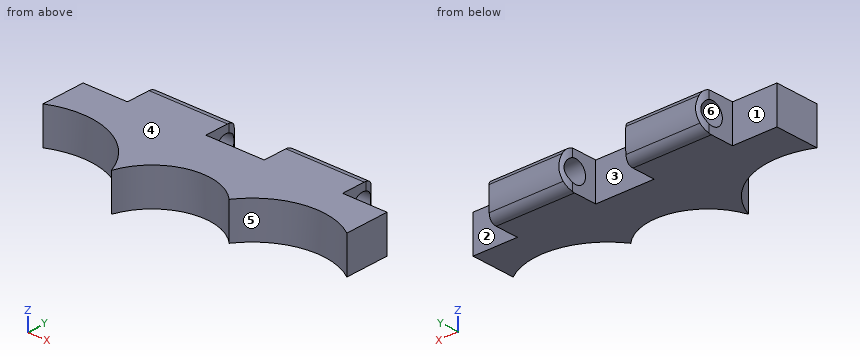
from build123d import *

# Parameters (mm, degrees)
SALIENTE_EXTRUIR1_DEPTH    = 5
CROQUIS5_R                 = 1.475
CORTAR_EXTRUIR3_DEPTH      = 10.6
CROQUIS10_R                = 1.475
CORTAR_EXTRUIR5_DEPTH      = 28.922395492
CORTAR_EXTRUIR6_DEPTH      = 38.568872355
CORTAR_EXTRUIR6_DEPTH_BACK = 38.568872355
REDONDEO5_R                = 1.5


with BuildPart() as part:
    # Croquis1 → Saliente-Extruir1 (new body)
    with BuildSketch(Plane.XY):
        with BuildLine():
            Line((-11.235063244, -0.5), (-5.235063244, -0.5))
            Line((-5.235063244, -0.5), (-5.235063244, 3))
            ThreePointArc((-5.235063244, 3), (-4.649276807, 4.414213562), (-3.235063244, 5))
            Line((-3.235063244, 5), (3.364936756, 5))
            ThreePointArc((3.364936756, 5), (4.779150318, 4.414213562), (5.364936756, 3))
            Line((5.364936756, 3), (5.364936756, -0.5))
            Line((5.364936756, -0.5), (13.264936756, -0.5))
            Line((13.264936756, -0.5), (13.264936756, 3))
            ThreePointArc((13.264936756, 3), (13.850723193, 4.414213562), (15.264936756, 5))
            Line((15.264936756, 5), (21.864936756, 5))
            ThreePointArc((21.864936756, 5), (23.279150318, 4.414213562), (23.864936756, 3))
            Line((23.864936756, 3), (23.864936756, -0.5))
            Line((23.864936756, -0.5), (29.864936756, -0.5))
            Line((29.864936756, -0.5), (29.864936756, -6.5))
            ThreePointArc((29.864936756, -6.5), (22.539313598, -4.979099508), (16.283876735, -9.083658268))
            ThreePointArc((16.283876735, -9.083658268), (8.876557279, -7.091468541), (3.364936756, -12.426188836))
            ThreePointArc((3.364936756, -12.426188836), (-2.643411058, -6.280927524), (-11.235063244, -6.5))
            Line((-11.235063244, -6.5), (-11.235063244, -0.5))
        make_face()
    extrude(amount=SALIENTE_EXTRUIR1_DEPTH)

    # Croquis5 → Cortar-Extruir3 (cut)
    with BuildSketch(Plane(origin=(23.864936756, 0, 0), x_dir=(0, 0, -1), z_dir=(1, 0, 0))):
        with Locations(Location((-2.5, 2.5, 0), (0, 0, 160.185071851))):
            Circle(CROQUIS5_R)
    extrude(amount=-CORTAR_EXTRUIR3_DEPTH, mode=Mode.SUBTRACT)

    # Croquis10 → Cortar-Extruir5 (cut, through all)
    with BuildSketch(Plane(origin=(5.364936756, 0, 0), x_dir=(0, 0, -1), z_dir=(1, 0, 0))):
        with Locations(Location((-2.5, 2.5, 0), (0, 0, 160.185071851))):
            Circle(CROQUIS10_R)
    extrude(amount=-CORTAR_EXTRUIR5_DEPTH, mode=Mode.SUBTRACT)

    # Croquis12 → Cortar-Extruir6 (cut, two sides: drawn at the far end of the back side and taken through both)
    with BuildSketch(Plane(origin=(23.864936756, 0, 0), x_dir=(0, 0, -1), z_dir=(1, 0, 0)).offset(-CORTAR_EXTRUIR6_DEPTH_BACK)):
        with BuildLine():
            Line((-35.945468922, -27.281986612), (-5.466117705, 3.197364605))
            ThreePointArc((-5.466117705, 3.197364605), (-2.561384811, 4.400544365), (0.343348083, 3.197364605))
            Line((0.343348083, 3.197364605), (30.8226993, -27.281986612))
            Line((30.8226993, -27.281986612), (30.8226993, 58.926637114))
            Line((30.8226993, 58.926637114), (-35.945468922, 58.926637114))
            Line((-35.945468922, 58.926637114), (-35.945468922, -27.281986612))
        make_face()
    extrude(amount=CORTAR_EXTRUIR6_DEPTH + CORTAR_EXTRUIR6_DEPTH_BACK, mode=Mode.SUBTRACT)

    # Redondeo5
    # the kernel refuses this fillet: 1.5 mm, written as the material it takes off along each edge
    with BuildSketch(Plane(origin=(7.90277719, 3.504212976, 0), x_dir=(0, -1, 0), z_dir=(-1, 0, 0)), Plane(origin=(26.40277719, 3.504212976, 0), x_dir=(0, -1, 0), z_dir=(-1, 0, 0))) as redondeo5_piece_1:
        with BuildLine():
            CenterArc((0.829424534, 1.5), REDONDEO5_R, 204.015661093, 65.984338907)
            ThreePointArc((-0.540726837, 0.889520499), (-0.298653835, 0.427562908), (0, 0))
            Line((0, 0), (0.829424534, 0))
        make_face()
    extrude(amount=15.675680868, mode=Mode.SUBTRACT)
    with BuildSketch(Plane(origin=(8.011290884, 3.59839975, 5), x_dir=(0, -1, 0), z_dir=(-1, 0, 0)), Plane(origin=(26.511290884, 3.59839975, 5), x_dir=(0, -1, 0), z_dir=(-1, 0, 0))) as redondeo5_piece_2:
        with BuildLine():
            CenterArc((0.872619886, -1.5), REDONDEO5_R, 90, 68.905299391)
            ThreePointArc((-0.526860355, -0.960134226), (-0.295570649, -0.462430475), (0, 0))
            Line((0, 0), (0.872619886, 0))
        make_face()
    extrude(amount=15.892708257, mode=Mode.SUBTRACT)


solid = part.part
Design review of the part built by this model. Coordinates are the model's own, in mm. Face numbers are marked on the shaded views. A direction names the side the tool comes from. Coordinates: 2 decimals unless noted, no trailing zeros. Loops run counter-clockwise (first coordinate to the right, second up) from the corner with the lowest first, then second, coordinate; pieces in that order, holes last. Notation, with made-up numbers: (42, 30.25) - (86, 30.25) arc R34 ccw to (86, 68.25) - close; hole circle Ø8 at (-11, -11.5). An arc over 180 degrees is marked (long way). Use CSV: the item, a comma, the result in double quotes. Start each with the question number.
1. Add section A-A on z = 1.7. Give the boundary of the cut face in (x, y), plus the area to 3 significant figures.
2. Mouldability with a two-part tool opening along Z and no side actions: class the marked faces 4, 5 and 6 as released by +Z, released by -Z, zero draft, split by the parting line, or undercut.
3. For the marked faces 1, 2 and 3, list the 3-axis set-ups (+Z, -Z, +X, -X, +Y, -Y) from which the entire face can be reached by the end or side of a thin tool; tool diameter is ignored.
4. Add section C-C on y = -8. Give the boundary of the cut face in (x, z).
5. Add section B-B on x = 18. Give the boundary of the cut face in (y, z) (3 decimals), plus the area to 3 significant figures.
6. Add section D-D on x = 0. Give the boundary of the cut face in (y, z) (3 decimals), plus the area to 3 significant figures.
7. To check wall thickness, follow probe 1 along Z at (x, y) = (1, 2.5) (3 decimals); probe 2 along Y at (x, z) = (-3, 1.7); probe 3 along X at (y, z) = (-8.5, 2.9). State the ranges of each line that lie inside material, in increasing order.
8. Clearance check with flat-ended pins moving along their axes: pin 1 (2.5 mm diameter, centred on y = 2.5, z = 2.5, fed in from -X); pin 2 (1.5 mm diameter, centred on x = 28, z = 1.5, fed in from +Y); pin 3 (1.8 mm diameter, centred on y = 1, z = 2.5, fed in from +X); pin 4 (3 mm diameter, centred on y = -9.5, z = 1, fed in from +X). State where each tip first meets the part, or that it passes through.
Resolved:
1,outline,"(-11.24, -6.5) arc R10.75 cw to (3.36, -12.43) arc R7.77 cw to (16.28, -9.08) arc R9.78 cw to (29.86, -6.5) - (29.86, -0.5) - (23.86, -0.5) - (23.86, 1.26) - (13.26, 1.26) - (13.26, -0.5) - (5.36, -0.5) - (5.36, 1.26) - (-5.24, 1.26) - (-5.24, -0.5) - (-11.24, -0.5) - close; (-5.09, 3.74) - (5.22, 3.74) arc R2 ccw to (4.88, 4.31) - (-4.75, 4.31) arc R2 ccw to start; (13.41, 3.74) - (23.72, 3.74) arc R2 ccw to (23.38, 4.31) - (13.75, 4.31) arc R2 ccw to start"
1,area,"311 mm2"
2,face 4,"released by +Z"
2,face 5,"zero draft"
2,face 6,"undercut"
3,face 1,"+Z, -Z, -X, +Y"
3,face 2,"+Z, -Z, +X, +Y"
3,face 3,"+Z, -Z, +Y"
4,outline,"(0.22, 0) - (6.74, 0) - (6.74, 5) - (0.22, 5) - close; (14.9, 0) - (17.14, 0) - (17.14, 5) - (14.9, 5) - close"
5,outline,"(-7.164, 0) - (2.675, 0) arc R1.5 ccw to (4.045, 0.89) arc R4.108 ccw to (4.125, 4.04) arc R1.5 ccw to (2.726, 5) - (-7.164, 5) - close; hole circle Ø2.95 at (2.5, 2.5)"
5,area,"49.4 mm2"
6,outline,"(-7.824, 0) - (2.675, 0) arc R1.5 ccw to (4.045, 0.89) arc R4.108 ccw to (4.125, 4.04) arc R1.5 ccw to (2.726, 5) - (-7.824, 5) - close; hole circle Ø2.95 at (2.5, 2.5)"
6,area,"52.7 mm2"
7,probe 1,"0 to 1.025, 3.975 to 5"
7,probe 2,"-6.14 to 1.26, 3.74 to 4.31"
7,probe 3,"0.77 to 6.03, 15.62 to 16.71"
8,pin 1,"through"
8,pin 2,"y = -0.5"
8,pin 3,"x = 23.86"
8,pin 4,"x = 17.14"
